```python
from build123d import *

# Parameters (mm, degrees)
SKETCH090_W     = 50.8
SKETCH090_H     = 27.7
PAD023_DEPTH    = 9.2
SKETCH091_W     = 6
SKETCH091_H     = 6
POCKET075_DEPTH = 10.2
SKETCH092_R     = 3
POCKET076_DEPTH = 11
POCKET077_DEPTH = 30.9
SKETCH094_R     = 2.85
POCKET078_DEPTH = 9.201
POCKET079_DEPTH = 9.201
SKETCH096_W     = 6.5
SKETCH096_H     = 6.5
PAD024_DEPTH    = 1.75
SKETCH097_W     = 5.2
SKETCH097_H     = 5.2
POCKET080_DEPTH = 1.75
FILLET004_R     = 10
FILLET005_R     = 15
FILLET006_R     = 1.5
SKETCH098_W     = 54.781057
SKETCH098_H     = 5.471817
POCKET081_DEPTH = 9.201
CHAMFER014_SIZE = 1.5
FILLET007_R     = 2


with BuildPart() as part:
    # Sketch090 → Pad023 (new body)
    with BuildSketch(Plane.XY):
        with Locations((0, -13.85)):
            Rectangle(SKETCH090_W, SKETCH090_H)
    extrude(amount=PAD023_DEPTH)

    # Sketch091 (on Face2 of Pad023) → Pocket075 (cut)
    with BuildSketch(Plane.XZ.offset(27.7)):
        with Locations((0, 4.5)):
            Rectangle(SKETCH091_W, SKETCH091_H)
    extrude(amount=-POCKET075_DEPTH, mode=Mode.SUBTRACT)

    # Sketch092 (on Face11 of Pocket075) → Pocket076 (cut)
    with BuildSketch(Plane.XZ.offset(17.5)):
        with Locations((0, 4.6)):
            Circle(SKETCH092_R)
    extrude(amount=-POCKET076_DEPTH, mode=Mode.SUBTRACT)

    # Sketch093 (on Face1 of Pocket076) → Pocket077 (cut)
    with BuildSketch(Plane(origin=(-25.4, 0, 0), x_dir=(0, -1, 0), z_dir=(-1, 0, 0))):
        Polygon((6.65774, 6.029261), (4.216094, 7.399795), (1.808354, 5.970534), (1.84226, 3.170739), (4.283906, 1.800205), (6.691646, 3.229466), align=None)
    extrude(amount=-POCKET077_DEPTH, mode=Mode.SUBTRACT)

    # Sketch094 (on Face4 of Pocket077) → Pocket078 (cut, through all)
    with BuildSketch(Plane.XY.offset(9.2)):
        with Locations((19.9, -17.515)):
            Circle(SKETCH094_R)
    extrude(amount=-POCKET078_DEPTH, mode=Mode.SUBTRACT)

    # Sketch095 (on Face4 of Pocket078) → Pocket079 (cut, through all)
    with BuildSketch(Plane.XY.offset(9.2)):
        Polygon((-7.4, -18.015), (-10.15, -13.25186), (-15.65, -13.25186), (-18.4, -18.015), (-15.65, -22.77814), (-10.15, -22.77814), align=None)
    extrude(amount=-POCKET079_DEPTH, mode=Mode.SUBTRACT)

    # Sketch096 (on Face5 of Pocket079) → Pad024 (join)
    with BuildSketch(Plane.XZ.offset(27.7)):
        with Locations((0, 4.6)):
            Rectangle(SKETCH096_W, SKETCH096_H)
    extrude(amount=PAD024_DEPTH)

    # Sketch097 (on Face29 of Pad024) → Pocket080 (cut)
    with BuildSketch(Plane.XZ.offset(29.45)):
        with Locations((0, 4.6)):
            Rectangle(SKETCH097_W, SKETCH097_H)
    extrude(amount=-POCKET080_DEPTH, mode=Mode.SUBTRACT)

    # Fillet004
    fillet004_edges = [part.edges().sort_by_distance(p)[0] for p in [
        (-25.4, -27.7, 4.6),
        (25.4, -27.7, 4.6),
    ]]
    fillet(fillet004_edges, radius=FILLET004_R)

    # Fillet005
    fillet005_edges = [part.edges().sort_by_distance(p)[0] for p in [
        (25.4, 0, 4.6),
    ]]
    fillet(fillet005_edges, radius=FILLET005_R)

    # Fillet006
    fillet006_edges = [part.edges().sort_by_distance(p)[0] for p in [
        (-25.4, 0, 4.6),
    ]]
    fillet(fillet006_edges, radius=FILLET006_R)

    # Sketch098 (on Face17 of Fillet006) → Pocket081 (cut, through all)
    with BuildSketch(Plane.XY.offset(9.2)):
        with Locations((-1.693186, -29.145549)):
            Rectangle(SKETCH098_W, SKETCH098_H)
    extrude(amount=-POCKET081_DEPTH, mode=Mode.SUBTRACT)

    # Chamfer014
    chamfer014_edges = [part.edges().sort_by_distance(p)[0] for p in [
        (17.05, -17.515, 9.2),
        (17.05, -17.515, 0),
    ]]
    chamfer(chamfer014_edges, length=CHAMFER014_SIZE)

    # Fillet007
    fillet007_edges = [part.edges().sort_by_distance(p)[0] for p in [
        (17.05, -17.515, 7.7),
        (17.05, -17.515, 1.5),
    ]]
    fillet(fillet007_edges, radius=FILLET007_R)


solid = part.part
```
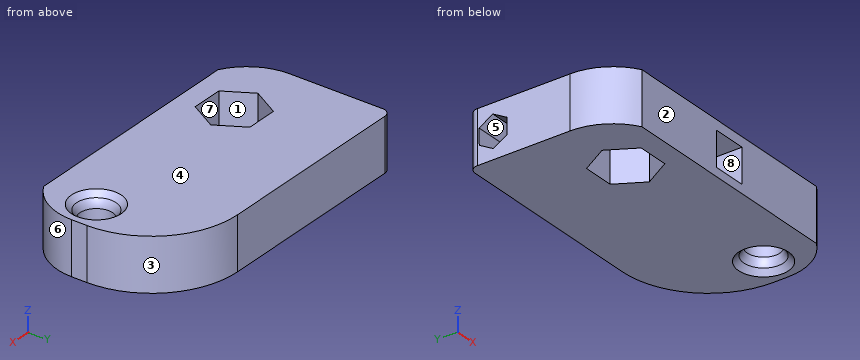
Input: part model. Units: mm. Frame: model coordinates. Face numbers are marked on the shaded views. A direction names the side the tool comes from. Round coordinates to 2 decimals unless told otherwise and drop trailing zeros. Order: outer loops, then holes, each group sorted by start corner. A loop starts at its lowest first (then second) coordinate and runs counter-clockwise, first axis right, second up. Notation, with made-up numbers: (-17.75, 40) - (18.25, 40) arc R21 ccw to (18.25, 57) - close; hole circle Ø7 at (51.25, 36). An arc over 180 degrees is marked (long way). One line per question, with ' | ' between items. Start each with the question number.
1) Ray query, probe 1 along Y at (x, z) = (-13, 5); probe 2 along Y at (x, z) = (-6.5, 5.5); probe 3 along X at (y, z) = (-16, 6.75). Return the intervals inside material, ascending.
2) Cut plane B-B, the plane x = 0. Return the cut outline in (y, z).
3) Cut plane C-C, the plane y = -23.25. Return the cut outline in (x, z), then the cut area to 3 significant figures.
4) Contact query for flat-ended pins moving along their axis: P1, Ø0.7, axis at x = -1, z = 7, coming from the -Y side; P2, Ø1.8, axis at y = -21.5, z = 5.5, coming from the +X side; P3, Ø7.5, axis at x = 19.9, y = -17.515, coming from the -Z side. Output: stop coordinate, or through.
5) Cut plane A-A, the plane z = 3.75. Return the cut outline in (x, y) (3 decimals).
6) Set-up query: the marked faces 4, 5, 6, 7 and 8. Return all of +Z, -Z, +X, -X, +Y, -Y with unobstructed straight access to the full face (end or side cutting, diameter ignored); none if empty.
7) Cut plane D-D, the plane y = -11. Return the cut outline in (x, z), then the cut area to 3 significant figures.
8) Pull-direction query (X, two-part tool) for the marked faces 1, 2 and 3; classes: +X half, -X half, draft (parallel to the pull), parting line (faces both ways), or undercut.
Worked out:
1) probe 1: y = -26.41 to -22.78, -13.25 to -6.67, -1.82 to 0 | probe 2: y = -26.41 to -6.66, -1.81 to 0 | probe 3: x = -25.4 to -17.24, -8.56 to -2.09, 2.09 to 17.49, 22.31 to 25.4
2) outline: (-26.41, 0) - (0, 0) - (0, 9.2) - (-26.41, 9.2) - (-26.41, 7.5) - (-17.5, 7.5) - (-17.5, 7.6) - (-6.5, 7.6) - (-6.5, 6.12) - (-4.22, 7.4) - (-1.81, 5.97) - (-1.84, 3.17) - (-4.28, 1.8) - (-6.5, 3.12) - (-6.5, 1.6) - (-17.5, 1.6) - (-17.5, 1.5) - (-26.41, 1.5) - close
3) outline: (-23.72, 0) - (23.72, 0) - (23.72, 9.2) - (-23.72, 9.2) - close; hole (-3, 1.5) - (3, 1.5) - (3, 7.5) - (-3, 7.5) - close | area: 400 mm^2
4) P1: stops at y = -6.5 | P2: stops at x = 24.97 | P3: stops at z = 0.6
5) outline: (-25.4, -17.7) arc R10 ccw to (-20.313, -26.41) - (-3, -26.41) - (-3, -17.5) - (-2.877, -17.5) - (-2.877, -6.685) - (-25.4, -6.685) - close; (-25.4, -1.835) - (5.5, -1.835) - (5.5, -6.685) - (2.877, -6.685) - (2.877, -17.5) - (3, -17.5) - (3, -26.41) - (20.313, -26.41) arc R10 ccw to (25.4, -17.7) - (25.4, -15) arc R15 ccw to (10.4, 0) - (-23.9, 0) arc R1.5 ccw to (-25.4, -1.5) - close; hole (-18.4, -18.015) - (-15.65, -22.778) - (-10.15, -22.778) - (-7.4, -18.015) - (-10.15, -13.252) - (-15.65, -13.252) - close; hole circle Ø5.7 at (19.9, -17.515)
6) face 4: +Z, +X, -X, +Y, -Y | face 5: -X | face 6: +Z, -Z, +X, -Y | face 7: +Z, -Z | face 8: -Y
7) outline: (-25.4, 0) - (24.86, 0) - (24.86, 9.2) - (-25.4, 9.2) - close; hole circle Ø6 at (0, 4.6) | area: 434 mm^2
8) face 1: undercut | face 2: draft | face 3: +X half
